The listing builds one solid part. Answer for the finished solid, in the listing's coordinates (mm). A direction names the side the tool comes from. Give positions to 0.01 mm unless a question says otherwise; leave off trailing zeros. Write each loop counter-clockwise with the first axis right and the second up, starting at its lowest first coordinate (ties: lowest second). Pieces come first, ordered by that corner, then holes. Notation, with made-up numbers: (22.25, 40) - (77.25, 40) arc R12 ccw to (77.25, 63) - close; hole circle Ø5 at (-34.5, 46). An arc over 180 degrees is marked (long way). Return JSON: item names as keys, results as strings.
from build123d import *

# Parameters (mm, degrees)
F0_R     = 2.475
F1_DEPTH = 11
F3_DEPTH = 15
F7_DEPTH = 10


with BuildPart() as f1:
    # F0 (on Front) → F1 (new body)
    with BuildSketch(Plane.XZ):
        Circle(F0_R)
    extrude(amount=F1_DEPTH)

    # F2 (on face) → F3 (join)
    with BuildSketch(Plane.XZ.offset(11)):
        with BuildLine():
            ThreePointArc((0.65, 2.2322914236), (0, 1.66842184), (-0.65, 2.2322914236))
            ThreePointArc((-0.65, 2.2322914236), (-1.3666007116, 1.8809645119), (-1.9221742584, 1.3080027219))
            ThreePointArc((-1.9221742584, 1.3080027219), (-1.5867634629, 0.5155707024), (-2.3238963511, 0.0716292507))
            ThreePointArc((-2.3238963511, 0.0716292507), (-2.2112064004, -0.7184645119), (-1.837969024, -1.4239012841))
            ThreePointArc((-1.837969024, -1.4239012841), (-0.9806737522, -1.3497816224), (-0.7862469313, -2.1880221121))
            ThreePointArc((-0.7862469313, -2.1880221121), (0, -2.325), (0.7862469313, -2.1880221121))
            ThreePointArc((0.7862469313, -2.1880221121), (0.9806737522, -1.3497816224), (1.837969024, -1.4239012841))
            ThreePointArc((1.837969024, -1.4239012841), (2.2112064004, -0.7184645119), (2.3238963511, 0.0716292507))
            ThreePointArc((2.3238963511, 0.0716292507), (1.5867634629, 0.5155707024), (1.9221742584, 1.3080027219))
            ThreePointArc((1.9221742584, 1.3080027219), (1.3666007116, 1.8809645119), (0.65, 2.2322914236))
        make_face()
    extrude(amount=F3_DEPTH)

    # F4 (on Right) → F5 (revolve)
    with BuildSketch(Plane.YZ):
        Polygon((0, 25.5), (0, 0), (75, 0), (75, 1.975), (39, 1.975), (39, 2.475), (33, 2.475), (33, 23.5), (30.5, 23.5), (28, 23.75), (25.5, 23.75), (23, 24), (20.5, 24), (18, 24.25), (15.5, 24.25), (13, 24.5), (10.5, 24.5), (8, 24.75), (5.5, 24.75), (3, 25), (0.5, 25), (0.5, 25.5), align=None)
    revolve(axis=Axis((0, 0, 0), (0, -1, 0)))

    # F6 (on face) → F7 (cut)
    with BuildSketch(Plane(origin=(0, 75, 0), x_dir=(-1, 0, 0), z_dir=(0, 1, 0))):
        with BuildLine():
            ThreePointArc((0.625, 1.8734993995), (0, 1.975), (-0.625, 1.8734993995))
            ThreePointArc((-0.625, 1.8734993995), (0, 1.5380774983), (0.625, 1.8734993995))
        make_face()
        with BuildLine():
            ThreePointArc((-1.8734993995, 0.625), (-1.975, 0), (-1.8734993995, -0.625))
            ThreePointArc((-1.8734993995, -0.625), (-1.5380774983, 0), (-1.8734993995, 0.625))
        make_face()
        with BuildLine():
            ThreePointArc((-0.625, -1.8734993995), (0, -1.975), (0.625, -1.8734993995))
            ThreePointArc((0.625, -1.8734993995), (0, -1.5380774983), (-0.625, -1.8734993995))
        make_face()
        with BuildLine():
            ThreePointArc((1.8734993995, -0.625), (1.975, 0), (1.8734993995, 0.625))
            ThreePointArc((1.8734993995, 0.625), (1.5380774983, 0), (1.8734993995, -0.625))
        make_face()
    extrude(amount=-F7_DEPTH, mode=Mode.SUBTRACT)


solid = f1.part
Item 1: A cutting plane is placed at A-A on y = 16.5. Determine the outline of the cut face in (x, z), then the cut area to 3 significant figures.
Answer below:
{"outline": "circle Ø48.5 at (0, 0)", "area": "1,850 mm²"}
Item 2: For faces 4 (the face through (-0.74, 35.96, 2.36)), 5 (the face through (0, -26, 0)), determine the directions among +Z, -Z, +X, -X, +Y, -Y from which every point of the face is accessible in a straight line to the end or side of a thin tool.
Answer below:
{"face 4": "+Y", "face 5": "+Z, -Z, +X, -X, -Y"}
Item 3: Consider L1, parallel to X at y = 43, z = -0.5; L2, parallel to Y at x = -19.5, z = -5.5; L3, parallel to X at y = 10, z = 1.5. Determine where each line is inside the solid, lowest interval first.
Answer below:
{"L1": "x = -1.91 to 1.91", "L2": "y = 0 to 33", "L3": "x = -24.5 to 24.5"}
Item 4: The mould has two halves that part along X. Classify faces 1 (the face through (18.8, 0.5, -16.9)), 2 (the face through (-7.1, 31.7, 22.4)), 3 (the face through (2, -11, 1)): +X half, -X half, draft (parallel to the pull), parting line (faces both ways), or undercut.
Answer below:
{"face 1": "draft", "face 2": "parting line", "face 3": "undercut"}
Item 5: Flat-ended cylindrical pins translate along their axes: P1, Ø1.5, axis at y = 9, z = 8.5, coming from the -X side; P2, Ø6, axis at x = 14, z = 10.5, coming from the +Y side; P3, Ø3, axis at y = -4.5, z = -3, coming from the +X side. Find the tip coordinate at first contact, or state that the pin passes through.
Answer below:
{"P1": "stops at x = -23.41", "P2": "stops at y = 33", "P3": "stops at x = 1.97"}
